```python
from build123d import *

# Parameters (mm, degrees)
F0_W          = 1016
F0_H          = 685.8
F1_DEPTH      = 38.1
F2_W          = 387.35
F2_H          = 463.55
F3_DEPTH      = 249.2375
F4_R          = 12.7
F5_DEPTH      = 127
F7_DEPTH      = 228.6
F7_DEPTH_BACK = 457.2


with BuildPart() as f1:
    # F0 (on Top) → F1 (new body)
    with BuildSketch(Plane.XY):
        with Locations((508, -342.9)):
            Rectangle(F0_W, F0_H)
    extrude(amount=F1_DEPTH)

    # F2 (on face) → F3 (join)
    with BuildSketch(Plane(origin=(0, 0, 0), x_dir=(1, 0, 0), z_dir=(0, 0, -1))):
        with Locations((504.825, 260.35)):
            Rectangle(F2_W, F2_H)
    extrude(amount=F3_DEPTH)

    # F4 (on face) → F5 (join)
    with BuildSketch(Plane(origin=(0, 0, 0), x_dir=(-1, 0, 0), z_dir=(0, 1, 0))):
        with Locations((-495.3, 19.05)):
            Circle(F4_R)
    extrude(amount=F5_DEPTH)

    # F6 (on face) → F7 (join, two sides)
    with BuildSketch(Plane.YZ.offset(1016)) as f7_sk:
        Polygon((-685.8, 12.7), (-685.8, 38.1), (-711.2, 38.1), (-711.2, 34.925), (-688.975, 34.925), (-688.975, 12.7), align=None)
        Polygon((25.4, 38.1), (0, 38.1), (0, 12.7), (3.175, 12.7), (3.175, 34.925), (25.4, 34.925), align=None)
    extrude(amount=F7_DEPTH)
    extrude(f7_sk.sketch, amount=-F7_DEPTH_BACK)


solid = f1.part
```
Geometry check sheet. Reference: the model listing, model coordinates, mm. A direction names the side the tool comes from. Give positions to 0.01 mm unless a question says otherwise; leave off trailing zeros. Write each loop counter-clockwise with the first axis right and the second up, starting at its lowest first coordinate (ties: lowest second). Pieces come first, ordered by that corner, then holes. Notation, with made-up numbers: (64.25, 58) -> (78.25, 58) arc R18 ccw to (78.25, 87) -> close; hole circle Ø11 at (-40, 44). An arc over 180 degrees is marked (long way). One line per question, with ' | ' between items.
Item 1: Access from +Z, -Z, +X, -X, +Y, -Y to the whole of each face (thin tool, end or side, straight path). Record for faces 1 (the flat face through (698.5, -257, -123)), 2 (the flat face through (558.8, 2, 31)), 3 (the flat face through (311.15, -257, -123)), 4 (the flat face through (1016, -348, 19)), 5 (the cylindrical face through (483.186, 62.611, 22.865)).
Determined:
face 1: -Z, +X, +Y, -Y | face 2: +Z, -Z, +Y | face 3: -Z, -X, +Y, -Y | face 4: +Z, -Z, +X | face 5: +Y
Item 2: Draft check along Y on faces 6 (the flat face through (1129, -685.8, 25)), 7 (the flat face through (1129, 0, 26)), 8 (the flat face through (502, -28.575, -123)), 9 (the flat face through (502, -492.125, -123)). Enter one of: released by +Y, released by -Y, zero draft, split by the parting line, or undercut.
Determined:
face 6: undercut | face 7: undercut | face 8: released by +Y | face 9: released by -Y
Item 3: Sectioned sample at A-A, the plane y = -186. Record the boundary of the cut face in (x, z), plus the area to 3 significant figures.
Determined:
outline: (0, 0) -> (311.15, 0) -> (311.15, -249.24) -> (698.5, -249.24) -> (698.5, 0) -> (1016, 0) -> (1016, 38.1) -> (0, 38.1) -> close | area: 135,000 mm^2
Item 4: Sectioned sample at C-C, the plane z = -40. Record the boundary of the cut face in (x, y) (3 decimals).
Determined:
outline: (311.15, -492.125) -> (698.5, -492.125) -> (698.5, -28.575) -> (311.15, -28.575) -> close
Item 5: Sectioned sample at D-D, the plane x = 934. Record the boundary of the cut face in (y, z) (3 decimals), plus the area to 3 significant figures.
Determined:
outline: (-711.2, 34.925) -> (-688.975, 34.925) -> (-688.975, 12.7) -> (-685.8, 12.7) -> (-685.8, 0) -> (0, 0) -> (0, 12.7) -> (3.175, 12.7) -> (3.175, 34.925) -> (25.4, 34.925) -> (25.4, 38.1) -> (-711.2, 38.1) -> close | area: 26,400 mm^2
Item 6: Scan lines: line 1 along X through (y, z) = (-282.5, -224.5); line 2 along Y through (x, z) = (339.5, -178.5) (3 decimals); line 3 along Y through (x, z) = (226, 20.5). Record each from-to range of solid material in increasing order.
Determined:
line 1: 311.15 to 698.5 | line 2: -492.125 to -28.575 | line 3: -685.8 to 0
Item 7: Depth check by flat-ended pin: pin 1 (1.5 mm diameter, centred on y = -451.5, z = -167.5, fed in from +X); pin 2 (24.5 mm diameter, centred on x = 847, z = 28, fed in from -Y); pin 3 (20.5 mm diameter, centred on y = 11.5, z = 29, fed in from -X); pin 4 (24.5 mm diameter, centred on x = 757, y = 16.5, fed in from -Z) (3 decimals). Enter the tip coordinate at first touch or a pass-through.
Determined:
pin 1: x = 698.5 | pin 2: y = -711.2 | pin 3: x = 482.6 | pin 4: z = 34.925
